Input: dimensioned drawing with shaded views. Units: mm. Origin: part minimum x, y, z. Coordinates: 2 decimals unless noted, no trailing zeros. Order: outer loops, then holes, each group sorted by start corner. A loop starts at its lowest first (then second) coordinate and runs counter-clockwise, first axis right, second up. Notation, with made-up numbers: (43, -28) - (71, -28) arc R22 cw to (71, 10) - close; hole circle Ø4 at (20, 8.25). An arc over 180 degrees is marked (long way). Answer as CSV lines item,"result". Start each with the question number.
Item 1: Draft query along Y for the marked faces 1, 2 and 3. Return one class per face: +Y half, -Y half, draft (parallel to the pull), parting line (faces both ways), or undercut.
Item 2: Section B-B (x = 0.75). Output: boundary loops of the cut face in (y, z) (1 decimal).
Item 3: Material intervals for line 1 along Y through (x, z) = (4.25, 11) (1 decimal); line 2 along Y through (x, z) = (2, 13.75) (1 decimal), sorted ascending.
Item 4: Section A-A (y = 11.5). Output: boundary loops of the cut face in (x, z), and give its area (3 significant figures).
Item 5: First-contact query: pin 1 (3 mm diameter, centred on x = 5.5, y = 18.5, fed in from -Z). Flat tip, straight axial feed; report the tip coordinate or a pass-through.
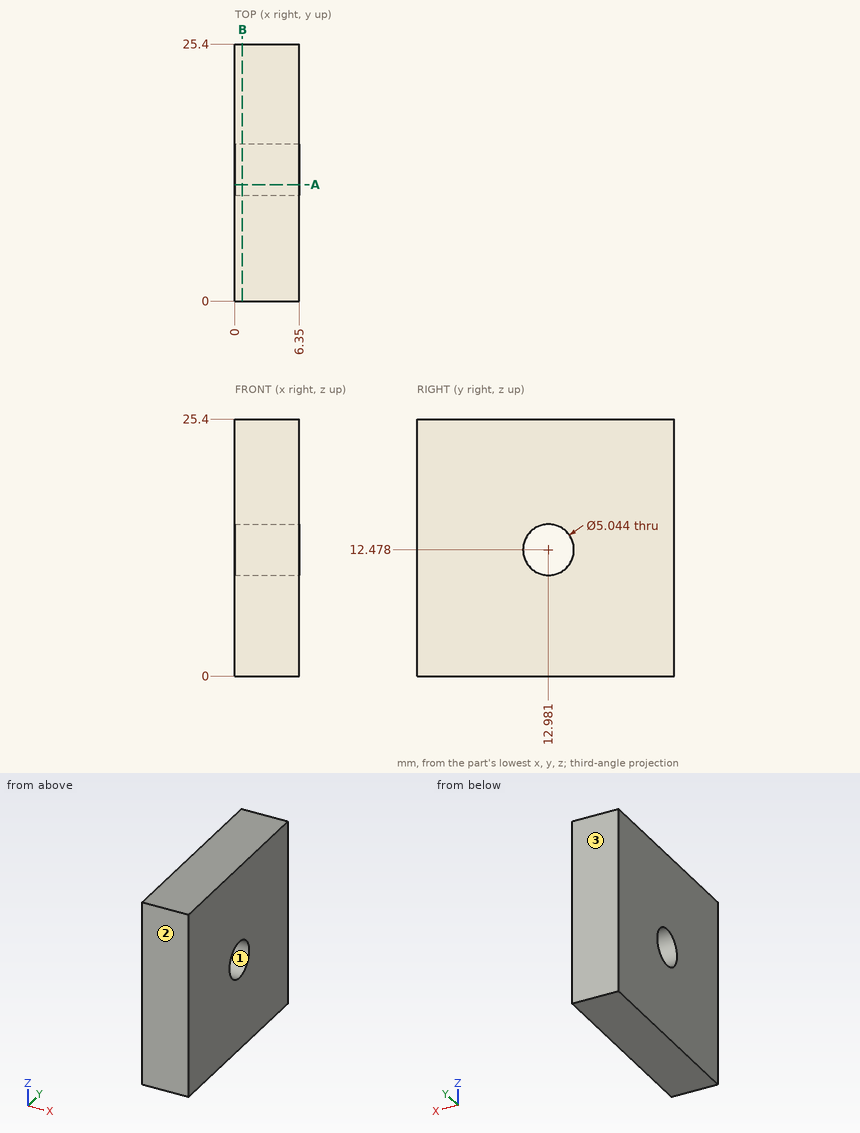
Determined:
1,face 1,"undercut"
1,face 2,"-Y half"
1,face 3,"+Y half"
2,outline,"(0, 0) - (25.4, 0) - (25.4, 25.4) - (0, 25.4) - close; hole circle Ø5 at (13, 12.5)"
3,line 1,"y = 0 to 10.9, 15 to 25.4"
3,line 2,"y = 0 to 10.8, 15.2 to 25.4"
4,outline,"(0, 0) - (6.35, 0) - (6.35, 10.44) - (0, 10.44) - close; (0, 14.52) - (6.35, 14.52) - (6.35, 25.4) - (0, 25.4) - close"
4,area,"135 mm^2"
5,pin 1,"stops at z = 0"
